Here's how the part is built. I have some questions about the finished solid (model axes, mm). A direction names the side the tool comes from. Round coordinates to 2 decimals unless told otherwise and drop trailing zeros. Loops run counter-clockwise (first coordinate to the right, second up) from the corner with the lowest first, then second, coordinate; pieces in that order, holes last. Notation, with made-up numbers: M 54,-20 L 66,-20 A20 cw 66,3 Z; hole C 15,-18.5 d3. An arc over 180 degrees is marked long. Use a Markdown table: item, result.
Autodesk Inventor part; units mm, degrees
ref_plane "YZ Plane" through (0, 0, 0) normal (1, 0, 0) x (0, 1, 0)
ref_plane "XZ Plane" through (0, 0, 0) normal (0, 1, 0) x (-1, 0, 0)
ref_plane "XY Plane" through (0, 0, 0) normal (0, 0, 1) x (1, 0, 0)
sketch "Sketch1" plane through (0, 0, 0) normal (0, 1, 0) x (-1, 0, 0)
  line L0 (0, 0) -> (5, 0)
  line L1 (5, 0) -> (5, -10)
  line L2 (5, -10) -> (0, -10)
  line L3 (0, -10) -> (0, 0)
  line L4 (-7.5, 20) -> (12.5, 20)
  line L5 (12.5, 20) -> (12.5, -30)
  line L6 (12.5, -30) -> (-7.5, -30)
  line L7 (-7.5, -30) -> (-7.5, 20)
  line L8 (-7.5, 20) -> (12.5, -30) construction
  line L9 (12.5, 20) -> (-7.5, -30) construction
  line L10 (12.5, -17.5) -> (12.5, 7.5)
  line L11 (12.5, 7.5) -> (-7.5, 7.5)
  line L12 (-7.5, 7.5) -> (-7.5, -17.5)
  line L13 (-7.5, -17.5) -> (12.5, -17.5)
  point P0 (2.5, -5)
  point P1 (-7.5, 7.5)
  dimension "d0" = 5
  dimension "d1" = 10
  dimension "d2" = 20
  dimension "d3" = 50
  dimension "d4" = 7.5
  dimension "d5" = 20
  dimension "d6" = 7.5
extrude "Extrusion1" add sketch "Sketch1" along normal blind 5
extrude "Extrusion2" add sketch "Sketch1" against normal blind 55 contours L11 L5 L13 L7
sketch "Sketch2" plane through (0, -55, 0) normal (0, -1, 0) x (1, 0, 0)
  line L0 (-12.5, 7.5) -> (-12.5, -17.5)
  line L1 (-12.5, -17.5) -> (7.5, -17.5)
  line L2 (7.5, -17.5) -> (7.5, 7.5)
  line L3 (7.5, 7.5) -> (-12.5, 7.5)
  line L4 (-5, 0) -> (0, 0)
  line L5 (0, 0) -> (0, -10)
  line L6 (0, -10) -> (-5, -10)
  line L7 (-5, -10) -> (-5, 0)
  line L8 (17.5, 17.5) -> (17.5, -27.5)
  line L9 (17.5, -27.5) -> (-22.5, -27.5)
  line L10 (-22.5, -27.5) -> (-22.5, 17.5)
  line L11 (-22.5, 17.5) -> (17.5, 17.5)
  line L12 (12.5, -22.5) -> (12.5, 12.5) construction
  line L13 (12.5, 12.5) -> (-17.5, 12.5) construction
  line L14 (-17.5, 12.5) -> (-17.5, -22.5) construction
  line L15 (-17.5, -22.5) -> (12.5, -22.5) construction
  circle A0 centre (12.5, 12.5) radius 1.5
  circle A1 centre (12.5, -22.5) radius 1.5
  circle A2 centre (-17.5, 12.5) radius 1.5
  circle A3 centre (-17.5, -22.5) radius 1.5
  dimension "d11" = 10
  dimension "d12" = 5
  dimension "d13" = 3
  dimension "d14" = 3
  dimension "d15" = 3
  dimension "d16" = 3
extrude "Extrusion3" add sketch "Sketch2" along normal blind 10 contours L8 L9 L10 L11
sketch "Sketch3" plane through (0, 5, 0) normal (0, 1, 0) x (1, 0, 0)
  line L0 (7.5, -20) -> (7.5, 30)
  line L1 (7.5, 30) -> (-12.5, 30)
  line L2 (-12.5, 30) -> (-12.5, -20)
  line L3 (-12.5, -20) -> (7.5, -20)
  line L4 (0, 0) -> (-5, 0)
  line L5 (-5, 0) -> (-5, 10)
  line L6 (-5, 10) -> (0, 10)
  line L7 (0, 10) -> (0, 0)
  line L8 (5, 15) -> (-10, 15)
  line L9 (-10, 15) -> (-10, -5)
  line L10 (-10, -5) -> (5, -5)
  line L11 (5, -5) -> (5, 15)
  dimension "d19" = 5
extrude "Extrusion4" cut sketch "Sketch3" against normal through all contours L11 L10 L9 L8
sketch "Sketch4" plane through (0, -55, 0) normal (0, -1, 0) x (1, 0, 0)
  line L0 (-10, 5) -> (5, 5)
  line L1 (5, 5) -> (5, -15)
  line L2 (5, -15) -> (-10, -15)
  line L3 (-10, -15) -> (-10, 5)
  line L4 (-12.5, 7.5) -> (-12.5, -17.5)
  line L5 (-12.5, -17.5) -> (7.5, -17.5)
  line L6 (7.5, -17.5) -> (7.5, 7.5)
  line L7 (7.5, 7.5) -> (-12.5, 7.5)
  point P0 (0, 0)
extrude "Extrusion5" add sketch "Sketch4" along normal blind 10
sketch "Sketch5" plane through (0, 5, 0) normal (0, 1, 0) x (1, 0, 0)
  line L0 (5, -5) -> (-10, -5)
  line L1 (-10, -5) -> (-10, 15)
  line L2 (-10, 15) -> (5, 15)
  line L3 (5, 15) -> (5, -5)
  line L4 (7.5, -20) -> (7.5, 30)
  line L5 (7.5, 30) -> (-12.5, 30)
  line L6 (-12.5, 30) -> (-12.5, -20)
  line L7 (-12.5, -20) -> (7.5, -20)
  circle A0 centre (-2.5, -15) radius 1.5
  circle A1 centre (-2.5, 25) radius 1.5
  point P0 (0, 0)
  dimension "d24" = 3
  dimension "d25" = 3
  dimension "d26" = 10
  dimension "d27" = 10
  dimension "d28" = 10
  dimension "d29" = 10
extrude "Extrusion6" cut sketch "Sketch5" against normal blind 10 contours A0 | A1
sketch "Sketch6" plane through (0, -65, 0) normal (0, -1, 0) x (1, 0, 0)
  line L0 (-10, 5) -> (5, 5)
  line L1 (5, 5) -> (5, -15)
  line L2 (5, -15) -> (-10, -15)
  line L3 (-10, -15) -> (-10, 5)
  line L4 (-22.5, 17.5) -> (-22.5, -27.5)
  line L5 (-22.5, -27.5) -> (17.5, -27.5)
  line L6 (17.5, -27.5) -> (17.5, 17.5)
  line L7 (17.5, 17.5) -> (-22.5, 17.5)
  circle A0 centre (12.5, 12.5) radius 1.5
  circle A1 centre (12.5, -22.5) radius 1.5
  circle A2 centre (-17.5, 12.5) radius 1.5
  circle A3 centre (-17.5, -22.5) radius 1.5
  point P0 (0, 0)
properties part number "select support V3_3DPrint"
1. Imagine slicing it at D-D, the plane x = 12.5. Write out the boundary of the cut face in (y, z).
Answer sheet:
| item | result |
|---|---|
| outline | M -65,-27.5 L -55,-27.5 L -55,-24 L -65,-24 Z; M -65,-21 L -55,-21 L -55,11 L -65,11 Z; M -65,14 L -55,14 L -55,17.5 L -65,17.5 Z |
2. Imagine slicing it at B-B, the plane x = -2.5. Write out the boundary of the cut face in (y, z).
Answer sheet:
| item | result |
|---|---|
| outline | M -65,-27.5 L -55,-27.5 L -55,-17.5 L 0,-17.5 L 0,-23.5 L 5,-23.5 L 5,-15 L -65,-15 Z; M -65,5 L 5,5 L 5,13.5 L 0,13.5 L 0,7.5 L -55,7.5 L -55,17.5 L -65,17.5 Z; M 0,-30 L 5,-30 L 5,-26.5 L 0,-26.5 Z; M 0,16.5 L 5,16.5 L 5,20 L 0,20 Z |
3. We'd pull the mould along Z, two halves only. Please class faces 5 (the face through (6, -65, -5)), 6 (the face through (-2, -60, -27.5)), 7 (the face through (11, -59.93, 12.43)): +Z half, -Z half, draft (parallel to the pull), parting line (faces both ways), or undercut.
Answer sheet:
| item | result |
|---|---|
| face 5 | draft |
| face 6 | -Z half |
| face 7 | undercut |
4. For pin 1 Ø8 at (x, z) = (-17, 0.5) entering from +Y; pin 2 Ø5 at (x, y) = (-8.5, -60.5) entering from -Z; pin 3 Ø3.5 at (x, z) = (-2.5, 15) entering from +Y; pin 4 Ø16 at (x, y) = (-1.5, -26) entering from +Z, each with a flat end and sliding along its axis, tell me the tip position at first contact or that it passes through.
Answer sheet:
| item | result |
|---|---|
| pin 1 | y = -55 |
| pin 2 | z = -27.5 |
| pin 3 | y = 5 |
| pin 4 | z = 7.5 |
5. Which directions (+Z, -Z, +X, -X, +Y, -Y) give clear straight access to the entire face, cutting with the end or side of a thin tool? Please do faces 1 (the face through (-1.114, 2.535, 15.575)), 2 (the face through (-2, -27, -17.5)), 3 (the face through (7.5, -25, -5)), 4 (the face through (-3, -60, 17.5)).
Answer sheet:
| item | result |
|---|---|
| face 1 | +Y |
| face 2 | -Z, +X, -X |
| face 3 | +Z, -Z, +X, +Y |
| face 4 | +Z, +X, -X, -Y |
6. Imagine slicing it at A-A, the plane z = 4. Write out the boundary of the cut face in (x, y), then the cut area to 3 significant figures.
Answer sheet:
| item | result |
|---|---|
| outline | M -22.5,-65 L -10,-65 L -10,5 L -12.5,5 L -12.5,-55 L -22.5,-55 Z; M 5,-65 L 17.5,-65 L 17.5,-55 L 7.5,-55 L 7.5,5 L 5,5 Z |
| area | 550 mm2 |
7. Imagine slicing it at C-C, the plane z = 15. Write out the boundary of the cut face in (x, y), then the cut area to 3 significant figures.
Answer sheet:
| item | result |
|---|---|
| outline | M -22.5,-65 L 17.5,-65 L 17.5,-55 L -22.5,-55 Z; M -12.5,0 L -4,0 L -4,5 L -12.5,5 Z; M -1,0 L 7.5,0 L 7.5,5 L -1,5 Z |
| area | 485 mm2 |
8. I need wall thicknesses on probe 1 along Z at (x, y) = (-17.5, -58); probe 2 along Z at (x, y) = (-2.5, 1.1); probe 3 along Z at (x, y) = (-1, -32). Which ranges of each line are inside material? Lowest first, please. Write a range as from..to.
Answer sheet:
| item | result |
|---|---|
| probe 1 | -27.5..-24, -21..11, 14..17.5 |
| probe 2 | -30..-26.5, -23.5..-15, 5..13.5, 16.5..20 |
| probe 3 | -17.5..-15, 5..7.5 |
